```python
from build123d import *

# Parameters (mm, degrees)
F0_W     = 19.05
F0_H     = 19.05
F0_W_2   = 15.875
F0_H_2   = 15.875
F1_DEPTH = 250
F3_DEPTH = 9.526
F4_DEPTH = 9.526


with BuildPart() as f1:
    # F0 (on Front) → F1 (new body)
    with BuildSketch(Plane.XZ):
        Rectangle(F0_W, F0_H)
        Rectangle(F0_W_2, F0_H_2, mode=Mode.SUBTRACT)
    extrude(amount=F1_DEPTH)

    # F2 (on Right) → F3 (cut, through all)
    with BuildSketch(Plane.YZ):
        Polygon((0, -9.525), (0, 9.525), (-19.05, -9.525), align=None)
        Polygon((-250, 9.525), (-250, -9.525), (-230.95, -9.525), align=None)
    extrude(amount=-F3_DEPTH, mode=Mode.SUBTRACT)

    # F2 (on Right) → F4 (cut, through all)
    with BuildSketch(Plane.YZ):
        Polygon((0, -9.525), (0, 9.525), (-19.05, -9.525), align=None)
        Polygon((-250, 9.525), (-250, -9.525), (-230.95, -9.525), align=None)
    extrude(amount=F4_DEPTH, mode=Mode.SUBTRACT)


solid = f1.part
```
Build history of the part. All positions in model axes, mm. A direction names the side the tool comes from. Round coordinates to 2 decimals unless told otherwise and drop trailing zeros. Loops run counter-clockwise (first coordinate to the right, second up) from the corner with the lowest first, then second, coordinate; pieces in that order, holes last.
Item 1: Two-plate mould, pull along X, no slides. Class faces 3 (the face through (0, -123, 9.525)), 4 (the face through (0, -123, 7.938)), 5 (the face through (-9.525, -123, 0)): released by +X, released by -X, zero draft, split by the parting line, or undercut.
Item 2: Which spindle directions (+Z, -Z, +X, -X, +Y, -Y) get a long thin tool onto all of the face, cutting with end or side? Do faces 1 (the face through (0, -123, -7.938)), 2 (the face through (-8.333, -9.392, 0.133)). Say none if no direction does.
Item 3: Saw through at B-B (z = -3). List the corners of the cut face in (x, y) (1 decimal), then the cut area to 3 significant figures.
Item 4: Drill centre lines: line 1 along Z through (x, y) = (-6.75, -217.5) (1 decimal); line 2 along Y through (x, z) = (8.25, 8) (3 decimals). Where is each one in solid material? Low to high.
Item 5: Saw through at C-C (y = -224). List the corners of the cut face in (x, z) (1 decimal).
Item 6: Pin check, flat tips, straight feed: P1, Ø8, axis at x = 5.5, z = 3.5, coming from the +Y side; P2, Ø1.5, axis at x = -2, z = -6, coming from the +Y side; P3, Ø4, axis at x = 0.5, z = 6.5, coming from the -Y side (3 decimals); P4, Ø8, axis at x = 6, z = 2.5, coming from the -Y side. Stop position of each tip, or through.
Worked answers:
1. face 3: zero draft
1. face 4: undercut
1. face 5: released by -X
2. face 1: +Y, -Y
2. face 2: -Z, +X, -X, +Y
3. outline: (-9.5, -237.5) - (-7.9, -237.5) - (-7.9, -12.5) - (-9.5, -12.5) - close; (7.9, -237.5) - (9.5, -237.5) - (9.5, -12.5) - (7.9, -12.5) - close
3. area: 714 mm2
4. line 1: z = -9.5 to -7.9, 7.9 to 9.5
4. line 2: y = -248.475 to -1.525
5. outline: (-9.5, -9.5) - (9.5, -9.5) - (9.5, 9.5) - (-9.5, 9.5) - close; hole (-7.9, -7.9) - (7.9, -7.9) - (7.9, 7.9) - (-7.9, 7.9) - close
6. P1: stops at y = -2.85
6. P2: passes through
6. P3: stops at y = -248.975
6. P4: stops at y = -246.47
